Check sheet for the modelled part. Datum: model origin and axes. Units: mm. A direction names the side the tool comes from. Give positions to 0.01 mm unless a question says otherwise; leave off trailing zeros. Order: outer loops, then holes, each group sorted by start corner. A loop starts at its lowest first (then second) coordinate and runs counter-clockwise, first axis right, second up.
Item 1: Sectioned sample at B-B on x = 46. Record the boundary of the cut face in (y, z), and give its area (3 significant figures).
Item 2: Material ranges on line 1 along Z through (x, y) = (78, 39.25); line 2 along Y through (x, z) = (27.5, -28.5); line 3 along Z through (x, y) = (80, 45), recorded low to high.
Item 3: Gauge pin test, flat ends, axial feed: P1, Ø5, axis at x = 53.5, y = 31.5, coming from the -Z side; P2, Ø4, axis at x = 36.5, z = 16.5, coming from the +Y side; P3, Ø3.5, axis at x = 52, z = -25, coming from the +Y side. Record the tip position at first contact, or that the pin passes through.
Item 4: Sectioned sample at C-C on y = 19. Record the boundary of the cut face in (x, z).
Item 5: Access from +Z, -Z, +X, -X, +Y, -Y to the whole of each face (thin tool, end or side, straight path). Record for faces 4 (the cylindrical face through (89.1, 40.92, 11.14)), 5 (the flat face through (69, 50, 0)), 6 (the cylindrical face through (71.22, 49.14, -11.1)), 7 (the flat face through (53, 49, 12)).
Item 6: Sectioned sample at A-A on x = 64.5. Record the boundary of the cut face in (y, z), and give its area (3 significant figures).
Item 7: Release check for a two-part mould opening along Y. For faces 1 (the flat face through (52, 25, 24)), 2 (the flat face through (52, 30, -18)), 3 (the flat face through (45.32, 52.6, 2.96)) record: released by +Y, released by -Y, zero draft, split by the parting line, or undercut.
Item 8: Sectioned sample at D-D on x = 74. Record the boundary of the cut face in (y, z).
from build123d import *

# Parameters (mm, degrees)
SKETCH1_R               = 10
BOSS_EXTRUDE1_DEPTH     = 90
CUT_EXTRUDE1_DEPTH      = 46
CUT_EXTRUDE1_DEPTH_BACK = 57
SKETCH3_W               = 32
SKETCH3_H               = 24
CUT_EXTRUDE2_DEPTH      = 20
BOSS_EXTRUDE2_DEPTH     = 32
SKETCH5_R               = 6
CUT_EXTRUDE3_DEPTH      = 78
FILLET3_R               = 3


with BuildPart() as part:
    # Sketch1 → Boss-Extrude1 (new body)
    with BuildSketch(Plane(origin=(0, 0, 0), x_dir=(0, 0, -1), z_dir=(1, 0, 0))):
        with BuildLine():
            Line((-30, 0), (30, 0))
            ThreePointArc((30, 0), (42.5, 12.5), (30, 25))
            Line((30, 25), (18, 25))
            Line((18, 25), (18, 35))
            Line((18, 35), (12, 35))
            Line((12, 35), (12, 70))
            Line((12, 70), (-12, 70))
            Line((-12, 70), (-12, 35))
            Line((-12, 35), (-18, 35))
            Line((-18, 35), (-18, 25))
            Line((-18, 25), (-30, 25))
            ThreePointArc((-30, 25), (-42.5, 12.5), (-30, 0))
        make_face()
        with Locations((0, 25)):
            Circle(SKETCH1_R, mode=Mode.SUBTRACT)
        Polygon((-6, 45), (6, 45), (0, 60), align=None, mode=Mode.SUBTRACT)
    extrude(amount=BOSS_EXTRUDE1_DEPTH)

    # Sketch2 → Cut-Extrude1 (cut, two sides)
    with BuildSketch(Plane.XY) as cut_extrude1_sk:
        Polygon((0, 0), (40.414518843, 70), (0, 70), align=None)
    extrude(amount=CUT_EXTRUDE1_DEPTH, mode=Mode.SUBTRACT)
    extrude(cut_extrude1_sk.sketch, amount=-CUT_EXTRUDE1_DEPTH_BACK, mode=Mode.SUBTRACT)

    # Sketch3 → Cut-Extrude2 (cut)
    with BuildSketch(Plane(origin=(0, 70, 0), x_dir=(1, 0, 0), z_dir=(0, 1, 0))):
        with Locations((74, 0)):
            Rectangle(SKETCH3_W, SKETCH3_H)
    extrude(amount=-CUT_EXTRUDE2_DEPTH, mode=Mode.SUBTRACT)

    # Sketch4 → Boss-Extrude2 (add)
    with BuildSketch(Plane(origin=(58, 0, 0), x_dir=(0, 0, -1), z_dir=(1, 0, 0))):
        Polygon((-6, 45), (-4, 50), (4, 50), (6, 45), align=None)
    extrude(amount=BOSS_EXTRUDE2_DEPTH)

    # Sketch5 → Cut-Extrude3 (cut)
    with BuildSketch(Plane(origin=(0, 50, 0), x_dir=(1, 0, 0), z_dir=(0, 1, 0))):
        with Locations((78, 0)):
            Circle(SKETCH5_R)
    extrude(amount=-CUT_EXTRUDE3_DEPTH, mode=Mode.SUBTRACT)

    # Fillet3
    fillet3_edges = [part.edges().sort_by_distance(p)[0] for p in [
        (90, 50, 0),
        (74, 50, 12),
        (58, 60, 12),
        (74, 50, -12),
        (58, 60, -12),
        (58, 70, 0),
        (90, 42.5, -12),
        (90, 42.5, 12),
    ]]
    fillet(fillet3_edges, radius=FILLET3_R)


solid = part.part
Report:
1. outline: (0, -30) arc R12.5 ccw to (25, -30) - (25, -18) - (35, -18) - (35, -12) - (70, -12) - (70, 12) - (35, 12) - (35, 18) - (25, 18) - (25, 30) arc R12.5 ccw to (0, 30) - close; hole circle Ø20 at (25, 0); hole (45, -6) - (60, 0) - (45, 6) - close
1. area: 2,790 mm2
2. line 1: z = -12 to -6, 6 to 12
2. line 2: y = 0 to 25
2. line 3: z = -12 to -5.66, 5.66 to 12
3. P1: stops at z = -18
3. P2: stops at y = 35
3. P3: stops at y = 25
4. outline: (10.97, -40.68) - (90, -40.68) - (90, -8) - (10.97, -8) - close; (10.97, 8) - (90, 8) - (90, 40.68) - (10.97, 40.68) - close
5. face 4: +Z, +X, +Y
5. face 5: +Z, -Z, +X, +Y
5. face 6: -Z, +X, +Y
5. face 7: +Z, +X, -X, +Y
6. outline: (0, -30) arc R12.5 ccw to (25, -30) - (25, -18) - (35, -18) - (35, -12) - (47, -12) arc R3 ccw to (50, -9) - (50, 9) arc R3 ccw to (47, 12) - (35, 12) - (35, 18) - (25, 18) - (25, 30) arc R12.5 ccw to (0, 30) - close; hole circle Ø20 at (25, 0)
6. area: 2,390 mm2
7. face 1: released by +Y
7. face 2: zero draft
7. face 3: undercut
8. outline: (0, -30) arc R12.5 ccw to (25, -30) - (25, -18) - (35, -18) - (35, -12) - (47, -12) arc R3 ccw to (50, -9) - (50, -4.47) - (33.94, -4.47) arc R10 cw to (16.06, -4.47) - (0, -4.47) - close; (0, 4.47) - (16.06, 4.47) arc R10 cw to (33.94, 4.47) - (50, 4.47) - (50, 9) arc R3 ccw to (47, 12) - (35, 12) - (35, 18) - (25, 18) - (25, 30) arc R12.5 ccw to (0, 30) - close
